Geometry check sheet. Reference: the model listing, model coordinates, mm. Round coordinates to 2 decimals unless told otherwise and drop trailing zeros. Write each loop counter-clockwise with the first axis right and the second up, starting at its lowest first coordinate (ties: lowest second). Pieces come first, ordered by that corner, then holes. Notation, with made-up numbers: M 35,67 L 73,67 A9 ccw 73,71 Z; hole C 22,8 d8. An arc over 180 degrees is marked long. Put each result on its own line as item: value. Start each with the question number.
(1) Material ranges on probe 1 along Z at (x, y) = (-0.05, 0.6); probe 2 along Z at (x, y) = (-1.1, -0.05); probe 3 along X at (y, z) = (-0.6, -1), recorded low to high.
(2) Section check C-C on z = -1. Record the cut outline in (x, y).
(3) Gauge pin test, flat ends, axial feed: pin 1 (1.5 mm diameter, centred on x = 1, z = -3.5, fed in from +Y); pin 2 (0.5 mm diameter, centred on x = -1, z = 1, fed in from +Y); pin 3 (1 mm diameter, centred on x = 0.5, z = -3, fed in from -Y). Record the tip position at first contact, or that the pin passes through.
(4) Section check A-A on y = 0. Record the cut outline in (x, z) (3 decimals), then the cut area to 3 significant figures.
(5) Mould release check, pull along X, two halves, no side actions. Record for faces 1 (the flat face through (0, 0, 0.4)), 2 (the cylindrical face through (1.617, 0.67, 0.496)), 3 (the flat face through (0, 0, -5.59)): pulls with the +X half, pulls with the -X half, needs draft (parallel to the pull), parting line crosses it, or undercut.
Autodesk Inventor part; units mm, degrees
ref_plane "YZ Plane" through (0, 0, 0) normal (1, 0, 0) x (0, 1, 0)
ref_plane "XZ Plane" through (0, 0, 0) normal (0, 1, 0) x (-1, 0, 0)
ref_plane "XY Plane" through (0, 0, 0) normal (0, 0, 1) x (1, 0, 0)
sketch "Esboço1" plane through (0, 0, 0) normal (0, 0, 1) x (1, 0, 0)
  circle A0 centre (0, 0) radius 1
  dimension "d0" = 2
extrude "Extrusão1" add sketch "Esboço1" against normal blind 5.59
sketch "Esboço2" plane through (0, 0, 0) normal (0, 0, 1) x (1, 0, 0)
  circle A0 centre (0, 0) radius 1.75
  dimension "d3" = 3.5
extrude "Extrusão2" add sketch "Esboço2" along normal blind 1
sketch "Esboço3" plane through (0, 0, 1) normal (0, 0, 1) x (1, 0, 0)
  line L0 (-0.25, -1.375) -> (0.25, -1.375)
  line L1 (0.25, -1.375) -> (0.25, 1.375)
  line L2 (0.25, 1.375) -> (-0.25, 1.375)
  line L3 (-0.25, 1.375) -> (-0.25, -1.375)
  line L4 (-0.25, -1.375) -> (0.25, 1.375) construction
  line L5 (0.25, -1.375) -> (-0.25, 1.375) construction
  line L6 (-1.375, -0.25) -> (1.375, -0.25)
  line L7 (1.375, -0.25) -> (1.375, 0.25)
  line L8 (1.375, 0.25) -> (-1.375, 0.25)
  line L9 (-1.375, 0.25) -> (-1.375, -0.25)
  line L10 (-1.375, -0.25) -> (1.375, 0.25) construction
  line L11 (1.375, -0.25) -> (-1.375, 0.25) construction
  point P0 (0, 0)
  point P1 (-0.25, 0.25)
  point P2 (-0.25, -0.25)
  point P3 (0.25, -0.25)
  point P4 (0.25, 0.25)
  dimension "d6" = 0.5
  dimension "d7" = 0.5
  dimension "d8" = 2.75
  dimension "d9" = 2.75
extrude "Extrusão3" cut sketch "Esboço3" against normal blind 0.6
thread "Rosca1"
fillet "Arredondamento2" radius 0.2 4 edges at (-0.25, 0.25, 0.7) (0.25, 0.25, 0.7) (-0.25, -0.25, 0.7) (0.25, -0.25, 0.7)
chamfer "Chanfro1" distance 0.25 angle 45 2 edges at (-1.75, 0, 1) (-1.75, 0, 0)
chamfer "Chanfro2" distance 0.2 angle 45 1 edges at (-1, 0, -5.59)
properties part number "Parafuso 2_2 mm" material "Liga de Nickel-Copper 400"
Answers follow:
1. probe 1: z = -5.59 to 0.4
1. probe 2: z = 0 to 0.4
1. probe 3: x = -0.8 to 0.8
2. outline: C 0,0 d2
3. pin 1: stops at y = 0.97
3. pin 2: stops at y = 1.48
3. pin 3: stops at y = -1
4. outline: M -1.75,0.25 L -1.5,0 L -1,0 L -1,-5.39 L -0.8,-5.59 L 0.8,-5.59 L 1,-5.39 L 1,0 L 1.5,0 L 1.75,0.25 L 1.75,0.75 L 1.5,1 L 1.375,1 L 1.375,0.4 L -1.375,0.4 L -1.375,1 L -1.5,1 L -1.75,0.75 Z
4. area: 12.9 mm^2
5. face 1: undercut
5. face 2: parting line crosses it
5. face 3: needs draft
